Geometry check sheet. Reference: the model listing, model coordinates, mm. Coordinates: 2 decimals unless noted, no trailing zeros. Order: outer loops, then holes, each group sorted by start corner. A loop starts at its lowest first (then second) coordinate and runs counter-clockwise, first axis right, second up. Notation, with made-up numbers: M 55,36 L 75,36 A21 ccw 75,68 Z; hole C -26,-39.75 d4. An arc over 180 degrees is marked long. One line per item, written item: value. Start each with the question number.
1) Sectioned sample at C-C, the plane y = -9. Enter the section's corners in (x, z), then the cut area to 3 significant figures.
2) Sectioned sample at A-A, the plane x = 0. Enter the section's corners in (y, z).
3) Thickness scan on L1, parallel to Y at x = 0, z = 20.75; L2, parallel to X at y = 1.5, z = 19.25; L3, parallel to Y at x = -8, z = 12.5. Record the ranges inside material, lowest first. Write a range as from..to.
4) Draft check along Y on faces 1 (the cylindrical face through (-14.13, 0.27, 15.21)), 2 (the flat face through (-9, 5, 30)), 3 (the cylindrical face through (-15.63, 11.99, 14.79)). Enter one of: pulls with the +Y half, pulls with the -Y half, needs draft (parallel to the pull), parting line crosses it, or undercut.
5) Go/stop test with flat-tipped pins: P1, Ø8, axis at x = -9, z = 25, coming from the -Y side; P2, Ø3, axis at y = -7.5, z = 18.5, coming from the +X side; P3, Ø8, axis at x = 13.5, z = 5.5, coming from the +Y side; P4, Ø3, axis at x = -8.5, y = -7, coming from the -Z side. Record where each tip stops, or that it passes through.
6) Sectioned sample at D-D, the plane z = 22.5. Enter the section's corners in (x, y).
Autodesk Inventor part; units mm, degrees
ref_plane "YZ Plane" through (0, 0, 0) normal (1, 0, 0) x (0, 1, 0)
ref_plane "XZ Plane" through (0, 0, 0) normal (0, 1, 0) x (-1, 0, 0)
ref_plane "XY Plane" through (0, 0, 0) normal (0, 0, 1) x (1, 0, 0)
sketch "草圖1" plane through (0, 0, 0) normal (0, 0, 1) x (1, 0, 0)
  line L0 (0, 27.58) -> (0, -27.58) construction
  line L1 (0, -27.58) -> (0, 27.58) construction
  line L2 (-27.58, 0) -> (27.58, 0) construction
  circle A0 centre (0, 0) radius 10
  circle A1 centre (0, 0) radius 16.179 construction
  circle A2 centre (0, 0) radius 19.7
  point P0 (16.179, 0)
  dimension "d1" = 32.358
  dimension "d0" = 20
  dimension "d2" = 39.4
extrude "擠出1" add sketch "草圖1" along normal blind 30
hole "孔1" at (16.179, 0, 0) direction (0, 0, 1) diameter 4.134 depth 61.1
pattern_circular "環形陣列1" count 4 over 360 about axis through (0, 0, 0) along (0, 0, 1) of "孔1"
properties part number "轉接版"
Final values:
1. outline: M -17.52,0 L -4.36,0 L -4.36,30 L -17.52,30 Z; M 4.36,0 L 17.52,0 L 17.52,30 L 4.36,30 Z
1. area: 790 mm^2
2. outline: M -19.7,0 L -18.25,0 L -18.25,30 L -19.7,30 Z; M -14.11,0 L -10,0 L -10,30 L -14.11,30 Z; M 10,0 L 14.11,0 L 14.11,30 L 10,30 Z; M 18.25,0 L 19.7,0 L 19.7,30 L 18.25,30 Z
3. L1: y = -19.7..-18.25, -14.11..-10, 10..14.11, 18.25..19.7
3. L2: x = -19.64..-17.6, -14.76..-9.89, 9.89..14.76, 17.6..19.64
3. L3: y = -18..-6, 6..18
4. face 1: undercut
4. face 2: needs draft
4. face 3: parting line crosses it
5. P1: stops at y = -19.05
5. P2: stops at x = 18.76
5. P3: stops at y = 17.26
5. P4: stops at z = 0
6. outline: C 0,0 d39.4; hole C -16.18,0 d4.13; hole C 0,0 d20; hole C 0,-16.18 d4.13; hole C 0,16.18 d4.13; hole C 16.18,0 d4.13
